Part print with two shaded views. Sizes in mm from the minimum x, y, z corner. Give positions to 0.01 mm unless a question says otherwise; leave off trailing zeros. Loops run counter-clockwise (first coordinate to the right, second up) from the corner with the lowest first, then second, coordinate; pieces in that order, holes last. Notation, with made-up numbers: (83, 48) -> (123, 48) arc R34 ccw to (123, 84) -> close; hole circle Ø4 at (36.5, 33). An arc over 180 degrees is marked (long way). One line per question, with ' | ' between items. Start each with the question number.
(1) Flat gauge pins, fed straight in: pin 1 Ø5.5 at (x, z) = (11.6, 11.6) entering from +Y; pin 2 Ø1.5 at (y, z) = (1, 2.5) entering from -X (1 decimal). Where does each tip first touch, or does it go through?
(2) Mould opens along Z. For the marked faces 1, 2 and 3 say: pulls with the +Z half, pulls with the -Z half, needs draft (parallel to the pull), parting line crosses it, or undercut.
(3) Slice it at A-A, the plane z = 11.6. Write the cut outline in (x, y).
(4) Slice it at C-C, the plane y = 3.8. Write the cut outline in (x, z).
(5) Drill centre lines: L1, parallel to X at y = 2, z = 9; L2, parallel to Z at x = 7.5, y = 2.75; L3, parallel to X at y = 2.55, z = 16.6. Where is each one in solid material? Low to high. Write a range as from..to.
(6) Slice it at B-B, the plane y = 0.5. Write the cut outline in (x, z).
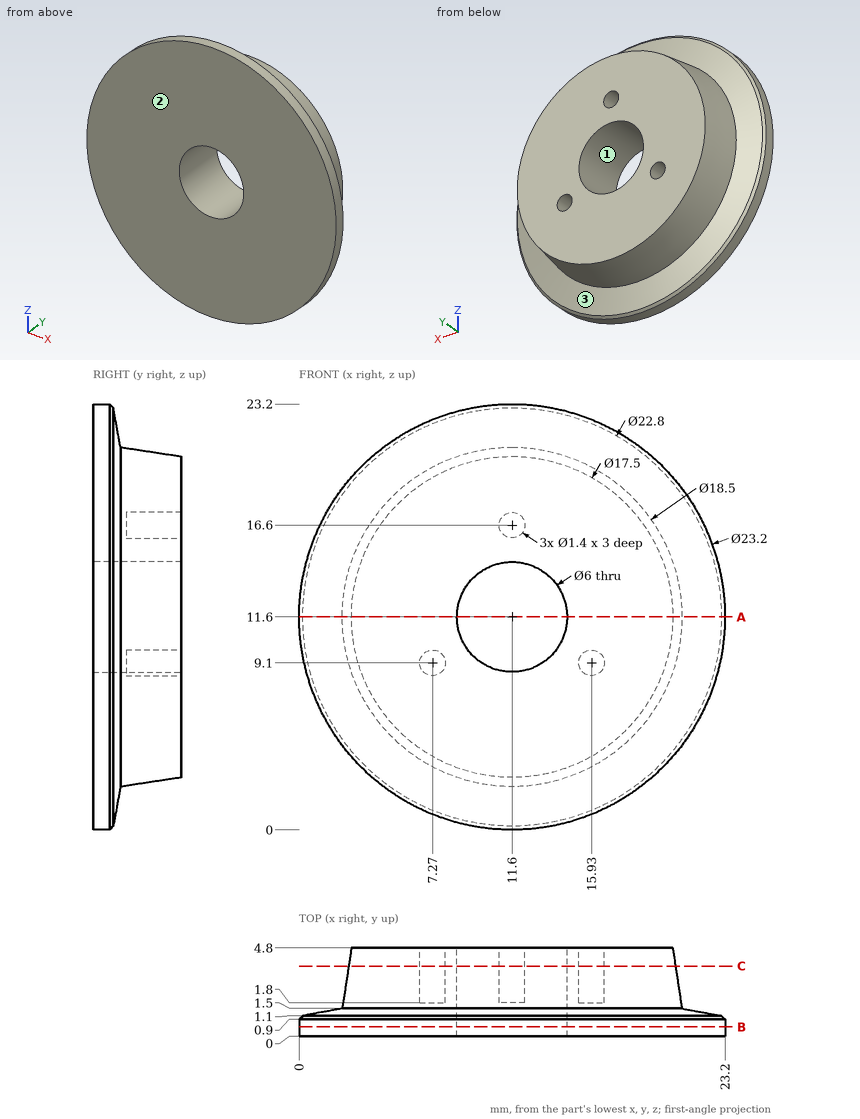
Final values:
1) pin 1: through | pin 2: x = 3.6
2) face 1: undercut | face 2: needs draft | face 3: parting line crosses it
3) outline: (0, 0) -> (8.6, 0) -> (8.6, 4.8) -> (2.85, 4.8) -> (2.35, 1.5) -> (0.2, 1.1) -> (0, 0.9) -> close; (14.6, 0) -> (23.2, 0) -> (23.2, 0.9) -> (23, 1.1) -> (20.85, 1.5) -> (20.35, 4.8) -> (14.6, 4.8) -> close
4) outline: circle Ø17.8 at (11.6, 11.6); hole circle Ø1.4 at (7.27, 9.1); hole circle Ø6 at (11.6, 11.6); hole circle Ø1.4 at (11.6, 16.6); hole circle Ø1.4 at (15.93, 9.1)
5) L1: 2.8..6.58, 7.96..10.1, 13.1..15.24, 16.62..20.4 | L2: 3.52..8.44, 9.76..19.68 | L3: 4.01..10.9, 12.3..19.19
6) outline: circle Ø23.2 at (11.6, 11.6); hole circle Ø6 at (11.6, 11.6)
